Geometry check sheet. Reference: the model listing, model coordinates, mm. Face numbers are marked on the shaded views. A direction names the side the tool comes from. Coordinates: 2 decimals unless noted, no trailing zeros. Order: outer loops, then holes, each group sorted by start corner. A loop starts at its lowest first (then second) coordinate and runs counter-clockwise, first axis right, second up. Notation, with made-up numbers: (14, 48.5) - (20, 48.5) arc R17 cw to (20, 56.5) - close; hole circle Ø10 at (50.5, 18). An arc over 180 degrees is marked (long way). Use CSV: the item, a comma, the result in double quotes. Start each with the question number.
1) Sectioned sample at D-D, the plane y = -57.5. Record the cut outline in (x, z), and give its area (3 significant figures).
2) Thickness scan on probe 1 along Z at (x, y) = (-5, 11); probe 2 along Y at (x, z) = (-3.5, 11.5); probe 3 along Y at (x, z) = (0.5, 2). Record the ranges inside material, lowest first. Write a range as [from, to].
3) Sectioned sample at C-C, the plane z = 26.75. Record the cut outline in (x, y), and give its area (3 significant figures).
4) Depth check by flat-ended pin: P1, Ø2, axis at x = 2, y = -51, coming from the -Z side; P2, Ø7, axis at y = -59.1, z = 21.87, coming from the +X side; P3, Ø3, axis at x = 11, y = -35.5, coming from the +Z side. Enter the tip coordinate at first touch or a pass-through.
5) Sectioned sample at A-A, the plane x = 0. Record the cut outline in (y, z).
6) Sectioned sample at B-B, the plane y = 0. Record the cut outline in (x, z).
7) Tool access check on the marked faces 1, 2, 3 and 4. Record the directions out of +Z, -Z, +X, -X, +Y, -Y that give a thin tool (end or side, any length) a straight path to the whole face; none if there is none.
from build123d import *

# Parameters (mm, degrees)
F0_W      = 30.6736361235
F0_H      = 84.459155798
F0_R      = 3.25
F1_DEPTH  = 3
F2_W      = 30.6736361235
F2_H      = 16.2
F3_DEPTH  = 3
F4_W      = 9.5
F4_H      = 16.2
F5_DEPTH  = 24
F6_W      = 3.5
F6_H      = 16.2452395454
F7_DEPTH  = 18
F9_DEPTH  = 25
F10_R     = 2.7291125689
F11_DEPTH = 20.0878180618


with BuildPart() as f1:
    # F0 (on Top) → F1 (new body)
    with BuildSketch(Plane.XY):
        Rectangle(F0_W, F0_H)
        Circle(F0_R, mode=Mode.SUBTRACT)
    extrude(amount=F1_DEPTH)

    # F2 (on face) → F3 (join)
    with BuildSketch(Plane.XY.offset(3)):
        with Locations((0, -34.129577899)):
            Rectangle(F2_W, F2_H)
    extrude(amount=F3_DEPTH)

    # F4 (on face) → F5 (join)
    with BuildSketch(Plane.XY.offset(6)):
        with Locations((0, -34.129577899)):
            Rectangle(F4_W, F4_H)
    extrude(amount=F5_DEPTH)

    # F6 (on face) → F7 (cut)
    with BuildSketch(Plane(origin=(0, -26.029577899, 0), x_dir=(-1, 0, 0), z_dir=(0, 1, 0))):
        with Locations((0.0963514363, 21.8773802273)):
            Rectangle(F6_W, F6_H)
    extrude(amount=-F7_DEPTH, mode=Mode.SUBTRACT)

    # F8 (on face) → F9 (join)
    with BuildSketch(Plane.XZ.offset(42.229577899)):
        Polygon((-1.8463514363, 30), (-4.75, 30), (-4.75, 12.3551307052), (-1.8463514363, 12.3551307052), (-1.8463514363, 13.7547604546), align=None)
        Polygon((4.75, 30), (1.6536485637, 30), (1.6536485637, 13.7547604546), (1.6540503129, 13.7547604546), (1.6540503129, 12.3551307052), (4.75, 12.3551307052), align=None)
    extrude(amount=F9_DEPTH)

    # F10 (on face) → F11 (cut, through all)
    with BuildSketch(Plane(origin=(-4.75, 0, 0), x_dir=(0, -1, 0), z_dir=(-1, 0, 0))):
        with BuildLine():
            Line((67.229577899, 30), (59.1030751607, 30))
            ThreePointArc((59.1030751607, 30), (64.8493803543, 27.6198024553), (67.229577899, 21.8734972618))
            Line((67.229577899, 21.8734972618), (67.229577899, 30))
        make_face()
        with BuildLine():
            Line((67.229577899, 12.3551307052), (67.229577899, 21.8734972618))
            ThreePointArc((67.229577899, 21.8734972618), (61.57093405, 14.1307768576), (52.4754527388, 17.1708737613))
            ThreePointArc((52.4754527388, 17.1708737613), (47.1597307325, 15.1731667126), (42.229577899, 12.3551307052))
            Line((42.229577899, 12.3551307052), (67.229577899, 12.3551307052))
        make_face()
        with Locations((59.1030751607, 21.8734972618)):
            Circle(F10_R)
        with BuildLine():
            Line((46.629577899, 30), (42.229577899, 30))
            Line((42.229577899, 30), (26.029577899, 30))
            Line((26.029577899, 30), (26.029577899, 28.4473763433))
            Line((26.029577899, 28.4473763433), (26.029577899, 15.8075261861))
            ThreePointArc((26.029577899, 15.8075261861), (38.3769053646, 22.0569473273), (51.7975745776, 25.4329505884))
            ThreePointArc((51.7975745776, 25.4329505884), (54.7952834092, 28.7642865475), (59.1030751607, 30))
            Line((59.1030751607, 30), (46.629577899, 30))
        make_face()
    extrude(amount=-F11_DEPTH, mode=Mode.SUBTRACT)


solid = f1.part
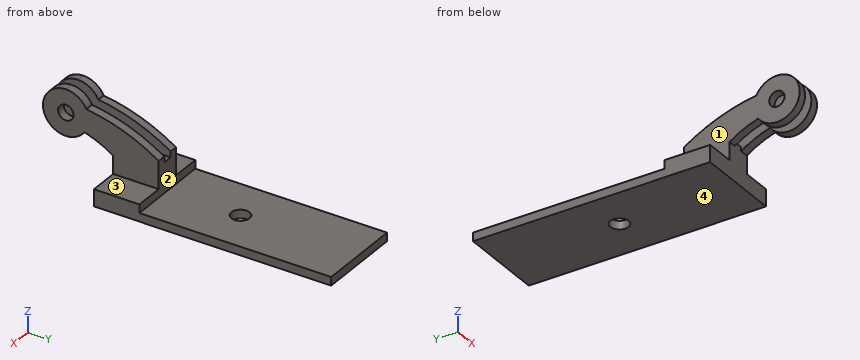
Evaluation:
1,outline,"(-4.75, 13.91) - (-1.85, 13.91) - (-1.85, 19.66) - (-4.75, 19.66) - close; (-4.75, 24.08) - (-1.85, 24.08) - (-1.85, 29.84) - (-4.75, 29.84) - close; (1.65, 13.91) - (4.75, 13.91) - (4.75, 19.66) - (1.65, 19.66) - close; (1.65, 24.08) - (4.75, 24.08) - (4.75, 29.84) - (1.65, 29.84) - close"
1,area,"69.1 mm²"
2,probe 1,"[0, 3]"
2,probe 2,"[-42.23, -26.03]"
2,probe 3,"[-42.23, -3.21], [3.21, 42.23]"
3,outline,"(-4.75, -65.6) - (-1.85, -65.6) - (-1.85, -52.6) - (-4.75, -52.6) - close; (1.65, -65.6) - (4.75, -65.6) - (4.75, -52.6) - (1.65, -52.6) - close"
3,area,"78.0 mm²"
4,P1,"z = 16.36"
4,P2,"x = 4.75"
4,P3,"z = 6"
5,outline,"(-42.23, 0) - (-3.25, 0) - (-3.25, 3) - (-26.03, 3) - (-26.03, 13.75) - (-42.23, 13.75) - close; (3.25, 0) - (42.23, 0) - (42.23, 3) - (3.25, 3) - close"
6,outline,"(-15.34, 0) - (-3.25, 0) - (-3.25, 3) - (-15.34, 3) - close; (3.25, 0) - (15.34, 0) - (15.34, 3) - (3.25, 3) - close"
7,face 1,"+Z, -X, +Y, -Y"
7,face 2,"+Z, +X, -X, +Y"
7,face 3,"+Z, +X, +Y, -Y"
7,face 4,"-Z, +X, -X, +Y, -Y"
